Part model, mm, in its own coordinate system. A direction names the side the tool comes from. Coordinates: 2 decimals unless noted, no trailing zeros. Loops run counter-clockwise (first coordinate to the right, second up) from the corner with the lowest first, then second, coordinate; pieces in that order, holes last. Notation, with made-up numbers: M 6.5,85 L 13.5,85 A27 cw 13.5,101 Z; hole C 63.25,71 d7. An arc over 180 degrees is marked long. Answer as a JSON object with one key per item and string values. Group by question number.
1. Saw through at D-D on y = 0. Write the cut outline in (x, z), then the cut area to 3 significant figures.
2. Saw through at A-A on x = -3.5. Write the cut outline in (y, z).
3. Drill centre lines: L1, parallel to Y at x = 13.5, z = -1.7; L2, parallel to Y at x = -16.75, z = 0.6; L3, parallel to Y at x = 18, z = -0.8. Where is each one in solid material? Low to high.
4. Mould opens along Y. For faces 4 (the face through (-2.114, -0.575, 0.042)), 5 (the face through (23, -13, 0)) say: released by +Y, released by -Y, zero draft, split by the parting line, or undercut.
5. Saw through at B-B on y = -8. Write the cut outline in (x, z), then the cut area to 3 significant figures.
6. 3-axis set-ups, long thin cutter, end or side, ignore diameter. For faces 1 (the face through (18, -2, 0)), 2 (the face through (4.1, 8, 0)), 3 (the face through (1, -3, -3)): which of +Z, -Z, +X, -X, +Y, -Y reach the whole face in a straight line?
7. Drop a flat-ended pin along its axis: pin 1 Ø0.7 at (y, z) = (6, 1) entering from +X. Give the stop position or say it passes through.
8. Saw through at C-C on x = 8.5. Write the cut outline in (y, z), then the cut area to 3 significant figures.
Autodesk Inventor part; units mm, degrees
sketch "Эскиз1" plane through (0, 0, 0) normal (0, 0, 1) x (1, 0, 0)
  line L0 (-20, -15) -> (20, -15)
  line L1 (20, -15) -> (20, 15)
  line L2 (20, 15) -> (-20, 15)
  line L3 (-20, 15) -> (-20, -15)
  line L4 (-20, -15) -> (20, 15) construction
  line L5 (20, -15) -> (-20, 15) construction
  point P0 (0, 0)
  dimension "d0" = 40
  dimension "d1" = 30
extrude "Выдавливание1" add sketch "Эскиз1" along normal mid plane 6
sketch "Эскиз2" plane through (0, 0, -3) normal (0, 0, -1) x (-1, 0, 0)
  circle A0 centre (16.75, 8) radius 1.25
  circle A1 centre (16.75, -8) radius 1.25
  point P0 (0, 0)
extrude "Выдавливание2" cut sketch "Эскиз2" against normal up to surface (6 mm away)
sketch "Эскиз3" plane through (20, -15, 3) normal (1, 0, 0) x (0, 0, -1)
  line L0 (0, 0) -> (0, 30)
  line L1 (6, 0) -> (6, 30)
  line L2 (0, 0) -> (6, 0)
  line L3 (6, 0) -> (6, 4)
  line L4 (6, 4) -> (0, 4)
  line L5 (0, 4) -> (0, 0)
  line L6 (0, 26) -> (6, 26)
  line L7 (6, 26) -> (6, 30)
  line L8 (6, 30) -> (0, 30)
  line L9 (0, 30) -> (0, 26)
  line L10 (6, 30) -> (6, 0)
  line L11 (0, 10) -> (6, 10)
  line L12 (6, 10) -> (6, 15)
  line L13 (0, 15) -> (0, 10)
  line L14 (0, 20) -> (6, 20)
  line L15 (6, 20) -> (6, 15)
  line L16 (0, 15) -> (0, 20)
  point P0 (3, 15)
  point P1 (0, 4)
  point P2 (0, 26)
  point P3 (6, 26)
  point P4 (6, 10)
  dimension "d6" = 4
  dimension "d7" = 4
extrude "Выдавливание3" add sketch "Эскиз3" along normal blind 3 contours L0 L4 L1 L2 | L0 L14 L1 L11 | L0 L8 L1 L6
sketch "Эскиз4" plane through (0, 0, 3) normal (0, 0, 1) x (1, 0, 0)
  line L0 (20, 6.55) -> (20, 9.45)
  line L1 (4.1, 9.45) -> (4.1, 6.55)
  line L2 (10.1, 10.8) -> (11.9, 10.8)
  line L3 (11.9, 5.2) -> (10.1, 5.2)
  line L4 (20, 9.45) -> (11.9, 9.45)
  line L5 (10.1, 9.45) -> (4.1, 9.45)
  line L6 (10.1, 5.2) -> (10.1, 6.55)
  line L7 (10.1, 9.45) -> (10.1, 10.8)
  line L8 (11.9, 10.8) -> (11.9, 9.45)
  line L9 (11.9, 6.55) -> (11.9, 5.2)
  line L10 (4.1, 6.55) -> (10.1, 6.55)
  line L11 (11.9, 6.55) -> (20, 6.55)
  line L12 (20, 5) -> (20, 11)
  line L13 (1.3154, 0) -> (2.8284, 0) construction
  line L14 (20, -6.55) -> (20, -9.45)
  line L15 (4.1, -9.45) -> (4.1, -6.55)
  line L16 (10.1, -10.8) -> (11.9, -10.8)
  line L17 (11.9, -5.2) -> (10.1, -5.2)
  line L18 (20, -9.45) -> (11.9, -9.45)
  line L19 (10.1, -9.45) -> (4.1, -9.45)
  line L20 (10.1, -5.2) -> (10.1, -6.55)
  line L21 (10.1, -9.45) -> (10.1, -10.8)
  line L22 (11.9, -10.8) -> (11.9, -9.45)
  line L23 (11.9, -6.55) -> (11.9, -5.2)
  line L24 (4.1, -6.55) -> (10.1, -6.55)
  line L25 (11.9, -6.55) -> (20, -6.55)
  point P0 (0, 0)
  point P1 (20, 0)
  point P2 (20, 8)
  dimension "d10" = 2.9
  dimension "d11" = 1.8
  dimension "d12" = 5.6
  dimension "d14" = 1.35
  dimension "d15" = 6
  dimension "d16" = 8.1
extrude "Выдавливание4" cut sketch "Эскиз4" against normal up to surface (6 mm away)
sketch "Эскиз5" plane through (0, 0, 3) normal (0, 0, 1) x (1, 0, 0)
  line L0 (-6, 2) -> (-10, 2)
  line L1 (-10, 2) -> (-10, -2)
  line L2 (-10, -2) -> (-6, -2)
  line L3 (-6, -2) -> (-6, 2)
  line L4 (-1, 2) -> (-1, -2)
  line L5 (-1, -2) -> (3, -2)
  line L6 (3, -2) -> (3, 2)
  line L7 (3, 2) -> (-1, 2)
  line L8 (7, 2) -> (7, -2)
  line L9 (11, 2) -> (7, 2)
  line L10 (7, -2) -> (11, -2)
  line L11 (11, -2) -> (11, 2)
  line L12 (16, 2) -> (16, -2)
  line L13 (20, 2) -> (16, 2)
  line L14 (16, -2) -> (20, -2)
  line L15 (20, -2) -> (20, 2)
  point P0 (0, 0)
extrude "Выдавливание5" cut sketch "Эскиз5" against normal up to surface (6 mm away)
sketch "Эскиз6" plane through (0, 0, 3) normal (0, 0, 1) x (1, 0, 0)
  circle A0 centre (-3.5, 0) radius 1.5
  circle A1 centre (13.5, 0) radius 1.5
  line L0 (-6, 2) -> (-6, -2)
  line L1 (-1, -2) -> (-1, 2)
  line L2 (11, 2) -> (11, -2)
  line L3 (16, -2) -> (16, 2)
  line L4 (-6, 0) -> (-1, 0) construction
  line L5 (11, 0) -> (16, 0) construction
  point P0 (0, 0)
  point P1 (-3.5, 0)
  point P2 (13.5, 0)
  dimension "d25" = 3
extrude "Выдавливание6" cut sketch "Эскиз6" against normal up to surface (6 mm away)
properties part number "крыло"
Outcome:
{
 "1": {"outline": "M -20,-3 L -10,-3 L -10,3 L -20,3 Z; M -6,-3 L -5,-3 L -5,3 L -6,3 Z; M -2,-3 L -1,-3 L -1,3 L -2,3 Z; M 3,-3 L 7,-3 L 7,3 L 3,3 Z; M 11,-3 L 12,-3 L 12,3 L 11,3 Z; M 15,-3 L 16,-3 L 16,3 L 15,3 Z; M 20,-3 L 23,-3 L 23,3 L 20,3 Z", "area": "126 mm²"},
 "2": {"outline": "M -15,-3 L -1.5,-3 L -1.5,3 L -15,3 Z; M 1.5,-3 L 15,-3 L 15,3 L 1.5,3 Z"},
 "3": {"L1": "y = -15 to -9.45, -6.55 to -1.5, 1.5 to 6.55, 9.45 to 15", "L2": "y = -15 to -9.25, -6.75 to 6.75, 9.25 to 15", "L3": "y = -15 to -9.45, -6.55 to -2, 2 to 6.55, 9.45 to 15"},
 "4": {"face 4": "undercut", "face 5": "zero draft"},
 "5": {"outline": "M -20,-3 L -18,-3 L -18,3 L -20,3 Z; M -15.5,-3 L 4.1,-3 L 4.1,3 L -15.5,3 Z", "area": "130 mm²"},
 "6": {"face 1": "+Z, -Z", "face 2": "+Z, -Z, +X", "face 3": "-Z, +X, -X, +Y, -Y"},
 "7": {"pin 1": "stops at x = 20"},
 "8": {"outline": "M -15,-3 L -9.45,-3 L -9.45,3 L -15,3 Z; M -6.55,-3 L -2,-3 L -2,3 L -6.55,3 Z; M 2,-3 L 6.55,-3 L 6.55,3 L 2,3 Z; M 9.45,-3 L 15,-3 L 15,3 L 9.45,3 Z", "area": "121 mm²"}
}
